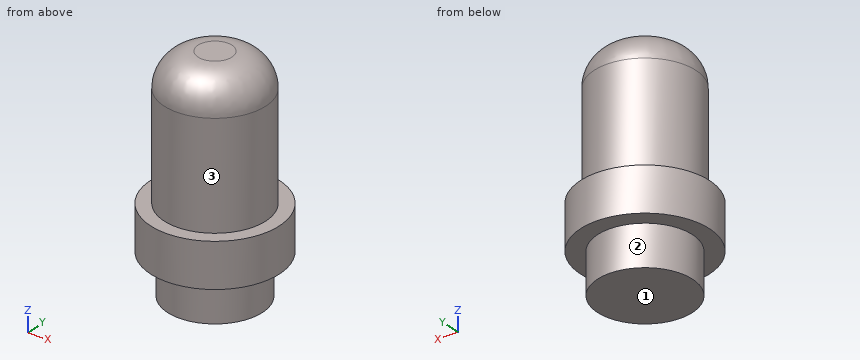
Autodesk Fusion 360 part; units mm, degrees
sketch "drawing" plane through (0, 0, 0) normal (1, 0, 0) x (0, 1, 0)
  line L0 (0, 4.1) -> (0.5, 4.1)
  line L1 (1.5, 3.1) -> (1.5, 0)
  line L2 (0, 0) -> (0, 4.1)
  line L3 (1.75, 0) -> (22.5, 0)
  line L4 (0, 1.75) -> (0, 22.5)
  arc A0 (1.5, 3.1) -> (0.5, 4.1) centre (0.5, 3.1) ccw
  line L5 (1.5, 0) -> (1.9, 0)
  line L6 (1.9, 0) -> (1.9, -1.3)
  line L7 (1.9, -1.3) -> (1.4, -1.3)
  line L8 (0, -1.3) -> (0, 0)
  line L9 (20, 0) -> (2.5, 0)
  line L10 (1.4, -1.3) -> (1.4, -2.5)
  line L11 (1.4, -2.5) -> (0, -2.5)
  line L12 (0, -2.5) -> (0, -1.3)
  dimension "d1" = 1.5
  dimension "d3" = 1
  dimension "d4" = 1.9
  dimension "d5" = 1.3
  dimension "d6" = 4.1
  dimension "d7" = 1.4
  dimension "d8" = 2.5
revolve "Revolve1" add sketch "drawing" angle 360 about axis through (0, 0, 0) along (0, 0, 1)
Read the model definition and answer for the solid it produces. Units are mm, in the model's axes. Face numbers are marked on the shaded views. A direction names the side the tool comes from. Round coordinates to 2 decimals unless told otherwise and drop trailing zeros. Write each loop counter-clockwise with the first axis right and the second up, starting at its lowest first coordinate (ties: lowest second). Pieces come first, ordered by that corner, then holes.
Q1. A tool of negligible diameter and unlimited length cuts with its end or side. For the marked faces 1, 2 and 3, from which of +Z, -Z, +X, -X, +Y, -Y can it reach the whole face along a straight path? Write none if from no direction.
Values:
face 1: -Z, +X, -X, +Y, -Y
face 2: -Z
face 3: +Z
Q2. Find section B-B on y = 1.6. Determine the outline of the cut face in (x, z), and give its area (3 significant figures).
Values:
outline: (-1.02, -1.3) - (1.02, -1.3) - (1.02, 0) - (-1.02, 0) - close
area: 2.66 mm2
Q3. Flat-ended cylindrical pins translate along their axes: P1, Ø1.1, axis at x = -1, y = -0.5, coming from the +Z side; P2, Ø1.5, axis at x = -0.5, z = 2.5, coming from the +Y side; P3, Ø1, axis at y = 1, z = -1, coming from the +X side; P4, Ø1, axis at y = 0.5, z = 0, coming from the +X side. Find the tip coordinate at first contact, or state that the pin passes through.
Values:
P1: stops at z = 4.1
P2: stops at y = 1.5
P3: stops at x = 1.83
P4: stops at x = 1.9
Q4. Straight lines are drawn through the part: line 1 (Z direction, x = -0.55, y = 1.6); line 2 (X direction, y = -0.05, z = -1.5); line 3 (Y direction, x = -1.25, z = -0.75). For each, find the intervals that lie inside material, in ascending order.
Values:
line 1: z = -1.3 to 0
line 2: x = -1.4 to 1.4
line 3: y = -1.43 to 1.43
Q5. Find section A-A on z = 2.5. Determine the outline of the cut face in (x, y).
Values:
outline: circle Ø3 at (0, 0)
